from build123d import *

# Parameters (mm, degrees)
SKETCH1_W            = 29
SKETCH1_H            = 6.75
BOSS_EXTRUDE10_DEPTH = 3.5
SKETCH1_16_R         = 0.291434634
BOSS_EXTRUDE15_DEPTH = 2
SKETCH1_17_W         = 29.75
SKETCH1_17_H         = 3
BOSS_EXTRUDE17_DEPTH = 35.2
SKETCH1_18_W         = 5
SKETCH1_18_H         = 1.912928139
SKETCH1_18_H_2       = 3
SKETCH1_18_H_3       = 1.837071861
BOSS_EXTRUDE20_DEPTH = 3.5
SKETCH2_W            = 25.95
SKETCH2_H            = 5
BOSS_EXTRUDE18_DEPTH = 1.75
FILLET1_R            = 2
FILLET3_R            = 2
FILLET2_R            = 4
SKETCH3_W            = 5.75
SKETCH3_H            = 1.125
CUT_EXTRUDE1_DEPTH   = 1.5
SKETCH4_R            = 1.85
BOSS_EXTRUDE19_DEPTH = 1.5
FILLET4_R            = 1.5


# Some blends are built 0.0001 mm under size
with BuildPart() as part:
    # Sketch1 → Boss-Extrude10 (new body)
    with BuildSketch(Plane.XY):
        with Locations((0, 3.375)):
            Rectangle(SKETCH1_W, SKETCH1_H)
        with BuildLine():
            Line((-12.052929028, 4.929746565), (0, 6.087071861))
            Line((0, 6.087071861), (12.052929028, 4.929746565))
            ThreePointArc((12.052929028, 4.929746565), (13.5, 3.337071861), (12.052929028, 1.744397157))
            Line((12.052929028, 1.744397157), (0, 0.587071861))
            Line((0, 0.587071861), (-12.052929028, 1.744397157))
            ThreePointArc((-12.052929028, 1.744397157), (-13.5, 3.337071861), (-12.052929028, 4.929746565))
        make_face(mode=Mode.SUBTRACT)
    extrude(amount=BOSS_EXTRUDE10_DEPTH)

    # Sketch1<16> → Boss-Extrude15 (add)
    # profile 1 of 9: a face of its own
    with BuildSketch(Plane.XY):
        with BuildLine():
            Line((-0.523286746, 6.036825735), (-12.052929028, 4.929746565))
            ThreePointArc((-12.052929028, 4.929746565), (-13.5, 3.337071861), (-12.052929028, 1.744397157))
            Line((-12.052929028, 1.744397157), (-0.523286746, 0.637317987))
            ThreePointArc((-0.523286746, 0.637317987), (-2.75, 3.337071861), (-0.523286746, 6.036825735))
        make_face()
        with Locations((-11.9, 3.337071861)):
            Circle(SKETCH1_16_R, mode=Mode.SUBTRACT)
        with Locations((-9.863185408, 3.337071861)):
            Circle(SKETCH1_16_R, mode=Mode.SUBTRACT)
        with Locations((-7.826370816, 3.337071861)):
            Circle(SKETCH1_16_R, mode=Mode.SUBTRACT)
    # profile 2 of 9: a face of its own
    with BuildSketch(Plane.XY):
        with Locations((-11.9, 3.337071861)):
            Circle(SKETCH1_16_R)
    # profile 3 of 9: a face of its own
    with BuildSketch(Plane.XY):
        with Locations((-7.826370816, 3.337071861)):
            Circle(SKETCH1_16_R)
    # profile 4 of 9: a face of its own
    with BuildSketch(Plane.XY):
        with Locations((-9.863185408, 3.337071861)):
            Circle(SKETCH1_16_R)
    # profile 5 of 9: a face of its own
    with BuildSketch(Plane.XY):
        with BuildLine():
            Line((0, 6.087071861), (-0.523286746, 6.036825735))
            ThreePointArc((-0.523286746, 6.036825735), (-2.75, 3.337071861), (-0.523286746, 0.637317987))
            Line((-0.523286746, 0.637317987), (0, 0.587071861))
            Line((0, 0.587071861), (0.523286746, 0.637317987))
            ThreePointArc((0.523286746, 0.637317987), (2.121501656, 1.587291668), (2.75, 3.337071861))
            ThreePointArc((2.75, 3.337071861), (2.121501656, 5.086852054), (0.523286746, 6.036825735))
            Line((0.523286746, 6.036825735), (0, 6.087071861))
        make_face()
    # profile 6 of 9: a face of its own
    with BuildSketch(Plane.XY):
        with BuildLine():
            Line((12.052929028, 4.929746565), (0.523286746, 6.036825735))
            ThreePointArc((0.523286746, 6.036825735), (2.121501656, 5.086852054), (2.75, 3.337071861))
            ThreePointArc((2.75, 3.337071861), (2.121501656, 1.587291668), (0.523286746, 0.637317987))
            Line((0.523286746, 0.637317987), (12.052929028, 1.744397157))
            ThreePointArc((12.052929028, 1.744397157), (13.5, 3.337071861), (12.052929028, 4.929746565))
        make_face()
        with Locations((7.826370816, 3.337071861)):
            Circle(SKETCH1_16_R, mode=Mode.SUBTRACT)
        with Locations((9.863185408, 3.337071861)):
            Circle(SKETCH1_16_R, mode=Mode.SUBTRACT)
        with Locations((11.9, 3.337071861)):
            Circle(SKETCH1_16_R, mode=Mode.SUBTRACT)
    # profile 7 of 9: a face of its own
    with BuildSketch(Plane.XY):
        with Locations((11.9, 3.337071861)):
            Circle(SKETCH1_16_R)
    # profile 8 of 9: a face of its own
    with BuildSketch(Plane.XY):
        with Locations((9.863185408, 3.337071861)):
            Circle(SKETCH1_16_R)
    # profile 9 of 9: a face of its own
    with BuildSketch(Plane.XY):
        with Locations((7.826370816, 3.337071861)):
            Circle(SKETCH1_16_R)
    extrude(amount=BOSS_EXTRUDE15_DEPTH)



with BuildPart() as body_2:
    # Sketch1<17> → Boss-Extrude17 (new body)
    with BuildSketch(Plane.XY):
        with Locations((34.375, 3.337071861)):
            Rectangle(SKETCH1_17_W, SKETCH1_17_H)
    extrude(amount=BOSS_EXTRUDE17_DEPTH)


with BuildPart() as part_1:
    add(part.part)

    add(body_2.part)  # Boss-Extrude20 merges body 2
    # Sketch1<18> → Boss-Extrude20 (add)
    with BuildSketch(Plane.XY):
        with Locations((17, 5.793535931)):
            Rectangle(SKETCH1_18_W, SKETCH1_18_H)
        with Locations((17, 3.337071861)):
            Rectangle(SKETCH1_18_W, SKETCH1_18_H_2)
        with Locations((17, 0.918535931)):
            Rectangle(SKETCH1_18_W, SKETCH1_18_H_3)
    extrude(amount=BOSS_EXTRUDE20_DEPTH)

    # Sketch2 → Boss-Extrude18 (add)
    with BuildSketch(Plane.XY.offset(35.2)):
        with Locations((6.525, 3.337071861)):
            Rectangle(SKETCH2_W, SKETCH2_H)
    extrude(amount=-BOSS_EXTRUDE18_DEPTH)

    # Fillet1
    # the kernel refuses this fillet: 2 mm, written as the material it adds along each edge
    with BuildSketch(Plane(origin=(19.5, 4.837071861, 33.45), x_dir=(1, 0, 0), z_dir=(0, 0, 1))) as fillet1_piece_1:
        with BuildLine():
            CenterArc((1.732050808, 2), FILLET1_R, 210, 60)
            Line((0, 1), (0, 0))
            Line((0, 0), (1.732050808, 0))
        make_face()
    extrude(amount=1.75)
    with BuildSketch(Plane(origin=(19.5, 4.837071861, 0), x_dir=(0, 1, 0), z_dir=(0, 0, 1))) as fillet1_piece_2:
        with BuildLine():
            CenterArc((2, -1.998103724), FILLET1_R, 92.495213733, 87.504786267)
            Line((0, -1.998103724), (0, 0))
            Line((0, 0), (1.912928139, 0))
        make_face()
    extrude(amount=3.5)
    with BuildSketch(Plane(origin=(19.5, 1.837071861, 33.45), x_dir=(1, 0, 0), z_dir=(0, 0, 1))) as fillet1_piece_3:
        with BuildLine():
            CenterArc((1.732050808, -2), FILLET1_R, 90, 60)
            Line((0, -1), (0, 0))
            Line((0, 0), (1.732050808, 0))
        make_face()
    extrude(amount=1.75)
    with BuildSketch(Plane(origin=(19.5, 1.837071861, 0), x_dir=(0, -1, 0), z_dir=(0, 0, 1))) as fillet1_piece_4:
        with BuildLine():
            CenterArc((2, 1.993352558), FILLET1_R, 180, 85.327274549)
            Line((0, 1.993352558), (0, 0))
            Line((0, 0), (1.837071861, 0))
        make_face()
    extrude(amount=3.5)

    # Fillet3
    fillet3_edges = [part_1.edges().sort_by_distance(p)[0] for p in [
        (19.5, 3.337071861, 3.5),
        (19.5, 3.337071861, 33.45),
    ]]
    fillet(fillet3_edges, radius=FILLET3_R)

    # Fillet2
    # the kernel refuses this fillet: 4 mm, written as the material it takes off along each edge
    with BuildSketch(Plane(origin=(-14.5, 6.75, -10), x_dir=(1, 0, 0), z_dir=(0, 0, 1)), Plane(origin=(-14.5, 0, -10), x_dir=(0, 1, 0), z_dir=(0, 0, 1))) as fillet2_piece_1:
        with BuildLine():
            CenterArc((FILLET2_R, -FILLET2_R), FILLET2_R, 90, 90)
            Line((0, -FILLET2_R), (0, 0))
            Line((0, 0), (FILLET2_R, 0))
        make_face()
    extrude(amount=23.5, mode=Mode.SUBTRACT)

    # Sketch3 → Cut-Extrude1 (cut)
    with BuildSketch(Plane.XY.offset(3.5)):
        with Locations((-0.102107464, 6.1875)):
            Rectangle(SKETCH3_W, SKETCH3_H)
        with Locations((-0.102107464, 0.5625)):
            Rectangle(SKETCH3_W, SKETCH3_H)
    extrude(amount=-CUT_EXTRUDE1_DEPTH, mode=Mode.SUBTRACT)

    # Sketch4 → Boss-Extrude19 (add)
    with BuildSketch(Plane.XY.offset(35.2)):
        with Locations((0.102107464, 3.375)):
            Circle(SKETCH4_R)
    extrude(amount=BOSS_EXTRUDE19_DEPTH)

    # Fillet4
    fillet4_edges = [part_1.edges().sort_by_distance(p)[0] for p in [
        (49.25, 4.837071861, 17.6),
        (49.25, 1.837071861, 17.6),
    ]]
    fillet(fillet4_edges, radius=FILLET4_R - 0.0001)  # a hair under: the kernel refuses the full size


solid = part_1.part
Could you check a few things on this model? Use its own coordinates, in mm. A direction names the side the tool comes from. Give positions to 0.01 mm unless a question says otherwise; leave off trailing zeros. Loops run counter-clockwise (first coordinate to the right, second up) from the corner with the lowest first, then second, coordinate; pieces in that order, holes last. Notation, with made-up numbers: (-17.5, 42) -> (34.5, 42) arc R30 ccw to (34.5, 65) -> close; hole circle Ø7 at (-3, 30.25). An arc over 180 degrees is marked (long way). Return JSON: item names as keys, results as strings.
Item 1: If we section it at D-D on x = -1: List the corners of the cut face in (y, z) for me.
Geometry results:
{"outline": "(0, 0) -> (6.75, 0) -> (6.75, 2) -> (0, 2) -> close; (0.84, 33.45) -> (5.84, 33.45) -> (5.84, 35.2) -> (4.86, 35.2) -> (4.86, 36.7) -> (1.89, 36.7) -> (1.89, 35.2) -> (0.84, 35.2) -> close"}
Item 2: If we section it at C-C on x = 38: List the corners of the cut face in (y, z) for me.
Geometry results:
{"outline": "(1.84, 0) -> (4.84, 0) -> (4.84, 35.2) -> (1.84, 35.2) -> close"}
Item 3: If we section it at A-A on x = 7: List the corners of the cut face in (y, z) for me.
Geometry results:
{"outline": "(0, 0) -> (6.75, 0) -> (6.75, 3.5) -> (5.41, 3.5) -> (5.41, 2) -> (1.26, 2) -> (1.26, 3.5) -> (0, 3.5) -> close; (0.84, 33.45) -> (5.84, 33.45) -> (5.84, 35.2) -> (0.84, 35.2) -> close"}
Item 4: I'm going to push flat-ended pins straight in: pin 1 (1 mm diameter, centred on y = 6.5, z = 3, fed in from -X); pin 2 (0.5 mm diameter, centred on y = 4.5, z = 34.5, fed in from -X); pin 3 (1 mm diameter, centred on y = 2.5, z = 15.5, fed in from -X). Where does each tip first touch, or does it pass through?
Geometry results:
{"pin 1": "stops at x = -12.83", "pin 2": "stops at x = -6.45", "pin 3": "stops at x = 19.5"}
Item 5: We'd pull the mould along Y, two halves only. Please class faces 4 (the cylindrical face through (48.82, 4.39, 17.85)), 5 (the cylindrical face through (-13.5, 3.3, 2.7)), 6 (the flat face through (11, 3, 0)): +Y half, -Y half, draft (parallel to the pull), parting line (faces both ways), or undercut.
Geometry results:
{"face 4": "+Y half", "face 5": "undercut", "face 6": "draft"}
Item 6: I need wall thicknesses on L1, parallel to Z at x = 3.5, y = 4.75; L2, parallel to X at y = 3.5, z = 31; L3, parallel to Y at x = 31, z = 33. Which ranges of each line are inside material? Lowest first, please. Write a range as from..to.
Geometry results:
{"L1": "z = 0..2, 33.45..35.2", "L2": "x = 19.5..49.24", "L3": "y = 1.84..4.84"}
Item 7: Which directions (+Z, -Z, +X, -X, +Y, -Y) give clear straight access to the entire face, cutting with the end or side of a thin tool? Please do faces 1 (the flat face through (19.5, 3, 18)), 2 (the flat face through (6, 5.837, 34)), 3 (the flat face through (7.35, 5.38, 2.74)).
Geometry results:
{"face 1": "-X, +Y, -Y", "face 2": "+Z, +X, -X, +Y", "face 3": "none"}
